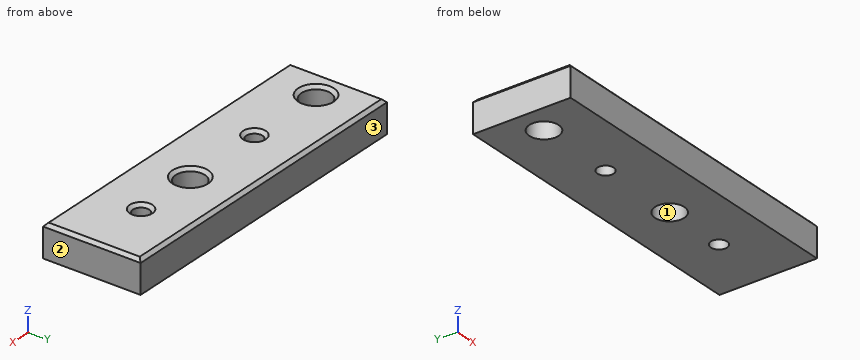
from build123d import *

# Parameters (mm, degrees)
F0_W     = 100
F0_H     = 30
F0_R     = 4.5
F0_R_2   = 2.5
F1_DEPTH = 10
F2_SIZE  = 1
F3_SIZE  = 1


with BuildPart() as f1:
    # F0 (on Top) → F1 (new body)
    with BuildSketch(Plane.XY):
        with Locations((-0.392441, 4.993296)):
            Rectangle(F0_W, F0_H)
        with Locations((-41.392441, 4.993296)):
            Circle(F0_R, mode=Mode.SUBTRACT)
        with Locations((-16.392441, 4.993296)):
            Circle(F0_R_2, mode=Mode.SUBTRACT)
        with Locations((9.607559, 4.993296)):
            Circle(F0_R, mode=Mode.SUBTRACT)
        with Locations((29.607559, 4.993296)):
            Circle(F0_R_2, mode=Mode.SUBTRACT)
    extrude(amount=F1_DEPTH)

    # F2
    f2_edges = [f1.edges().sort_by_distance(p)[0] for p in [
        (-0.392441, -10.006704, 10),
        (-50.392441, 4.993296, 10),
        (-0.392441, 19.993296, 10),
        (49.607559, 4.993296, 10),
    ]]
    chamfer(f2_edges, length=F2_SIZE)

    # F3
    f3_edges = [f1.edges().sort_by_distance(p)[0] for p in [
        (-45.892441, 4.993296, 10),
        (-18.892441, 4.993296, 10),
        (5.107559, 4.993296, 10),
        (27.107559, 4.993296, 10),
    ]]
    chamfer(f3_edges, length=F3_SIZE)


solid = f1.part
Read the model definition and answer for the solid it produces. Units are mm, in the model's axes. Face numbers are marked on the shaded views. Coordinates: 2 decimals unless noted, no trailing zeros. Loops run counter-clockwise (first coordinate to the right, second up) from the corner with the lowest first, then second, coordinate; pieces in that order, holes last. Notation, with made-up numbers: (19.5, 1.5) -> (54.5, 1.5) arc R24 cw to (54.5, 35.5) -> close; hole circle Ø5 at (76, 12). An arc over 180 degrees is marked (long way). Answer in a Markdown table with one row per item.
Item 1: A cutting plane is placed at A-A on z = 1.5. Determine the outline of the cut face in (x, y).
Returned:
| item | result |
|---|---|
| outline | (-50.39, -10.01) -> (49.61, -10.01) -> (49.61, 19.99) -> (-50.39, 19.99) -> close; hole circle Ø9 at (-41.39, 4.99); hole circle Ø5 at (-16.39, 4.99); hole circle Ø9 at (9.61, 4.99); hole circle Ø5 at (29.61, 4.99) |
Item 2: Straight lines are drawn through the part: line 1 along X through (y, z) = (4, 0.5); line 2 along X through (y, z) = (2, 2.75); line 3 along Y through (x, z) = (8, 3). For each, find the intervals that lie inside material, in ascending order. Write a range as [from, to].
Returned:
| item | result |
|---|---|
| line 1 | x = [-50.39, -45.78], [-37, -18.69], [-14.1, 5.22], [14, 27.31], [31.9, 49.61] |
| line 2 | x = [-50.39, -44.75], [-38.03, 6.25], [12.97, 49.61] |
| line 3 | y = [-10.01, 0.79], [9.2, 19.99] |
Item 3: Each of these flat-tipped pins is pushed along its axis until it touches: P1, Ø8, axis at x = 29.61, y = 4.99, coming from the -Z side; P2, Ø4, axis at x = -16.39, y = 4.99, coming from the +Z side. Where does it stop, or does it pass through?
Returned:
| item | result |
|---|---|
| P1 | stops at z = 0 |
| P2 | passes through |
Item 4: For a pull along Y with two mould halves and no side action, classify the marked faces 1, 2 and 3 as released by +Y, released by -Y, zero draft, split by the parting line, or undercut.
Returned:
| item | result |
|---|---|
| face 1 | undercut |
| face 2 | zero draft |
| face 3 | released by +Y |
